from build123d import *

# Parameters (mm, degrees)
SKETCH_1_W          = 45
SKETCH_1_H          = 51
EXTRUDE_1_DEPTH     = 30
SKETCH_2_W          = 27
SKETCH_2_H          = 48
CUT_EXTRUDE_1_DEPTH = 60.793394284
SKETCH_3_R          = 1.5
SKETCH_3_W          = 26
SKETCH_3_H          = 17
CUT_EXTRUDE_2_DEPTH = 61.911821513
FILLET_1_R          = 3
SKETCH_4_R          = 13
SKETCH_4_R_2        = 2
CUT_EXTRUDE_3_DEPTH = 30
FILLET_2_R          = 10
FILLET_3_R          = 5


with BuildPart() as part:
    # 草图1 → 凸台-拉伸1 (new body)
    with BuildSketch(Plane.XY):
        Rectangle(SKETCH_1_W, SKETCH_1_H)
    extrude(amount=EXTRUDE_1_DEPTH)

    # 草图2 → 切除-拉伸1 (cut, through all)
    with BuildSketch(Plane(origin=(22.5, 0, 0), x_dir=(0, 0, -1), z_dir=(1, 0, 0))):
        with Locations((-16.5, 1.5)):
            Rectangle(SKETCH_2_W, SKETCH_2_H)
    extrude(amount=-CUT_EXTRUDE_1_DEPTH, mode=Mode.SUBTRACT)

    # 草图3 → 切除-拉伸2 (cut, through all)
    with BuildSketch(Plane(origin=(0, -22.5, 0), x_dir=(1, 0, 0), z_dir=(0, 1, 0))):
        with Locations(Location((-17.5, -8, 0), (0, 0, 270))):
            Circle(SKETCH_3_R)
        with Locations(Location((-17.5, -25, 0), (0, 0, 270))):
            Circle(SKETCH_3_R)
        with Locations(Location((17.5, -25, 0), (0, 0, 90))):
            Circle(SKETCH_3_R)
        with Locations(Location((17.5, -8, 0), (0, 0, 90))):
            Circle(SKETCH_3_R)
        with Locations((0, -16.5)):
            Rectangle(SKETCH_3_W, SKETCH_3_H)
    extrude(amount=-CUT_EXTRUDE_2_DEPTH, mode=Mode.SUBTRACT)

    # 圆角1
    fillet_1_edges = [part.edges().sort_by_distance(p)[0] for p in [
        (13, -24, 8),
        (13, -24, 25),
        (-13, -24, 25),
        (-13, -24, 8),
    ]]
    fillet(fillet_1_edges, radius=FILLET_1_R)

    # 草图4 → 切除-拉伸3 (cut)
    with BuildSketch(Plane.XY.offset(3)):
        with Locations((0, 3)):
            Circle(SKETCH_4_R)
        with Locations((12.374368671, 15.374368671)):
            Circle(SKETCH_4_R_2)
        with Locations((-12.374368671, 15.374368671)):
            Circle(SKETCH_4_R_2)
        with Locations((-12.374368671, -9.374368671)):
            Circle(SKETCH_4_R_2)
        with Locations((12.374368671, -9.374368671)):
            Circle(SKETCH_4_R_2)
    extrude(amount=-CUT_EXTRUDE_3_DEPTH, mode=Mode.SUBTRACT)

    # 圆角2
    fillet_2_edges = [part.edges().sort_by_distance(p)[0] for p in [
        (-22.5, 25.5, 1.5),
        (22.5, 25.5, 1.5),
    ]]
    fillet(fillet_2_edges, radius=FILLET_2_R)

    # 圆角3
    fillet_3_edges = [part.edges().sort_by_distance(p)[0] for p in [
        (-22.5, -24, 30),
        (22.5, -24, 30),
    ]]
    fillet(fillet_3_edges, radius=FILLET_3_R)


solid = part.part
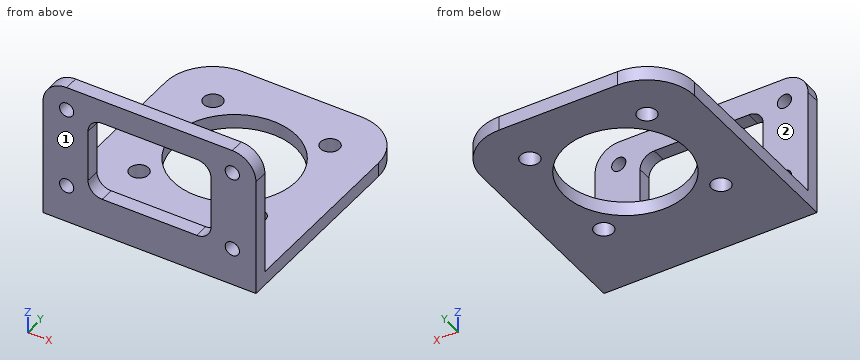
Can you work these out from the model? Positions are in its coordinate system, mm. Face numbers are marked on the shaded views. A direction names the side the tool comes from. Give positions to 0.01 mm unless a question says otherwise; leave off trailing zeros. Order: outer loops, then holes, each group sorted by start corner. A loop starts at its lowest first (then second) coordinate and runs counter-clockwise, first axis right, second up. Notation, with made-up numbers: M 31,16.5 L 83,16.5 A28 ccw 83,37.5 Z; hole C 55.5,24 d2. An arc over 180 degrees is marked long. Use one line per item in the form item = value. Start each with the question number.
Item 1: If we section it at C-C (z = 14.25): Write out the boundary of the cut face in (x, y).
Item 2: If we section it at B-B (y = 8): Write out the boundary of the cut face in (x, z), then the cut area to 3 significant figures.
Item 3: Will these pins go through, and if not, where does the flat tip stop? pin 1 Ø3 at (x, y) = (12.37, 15.37) entering from +Z; pin 2 Ø4 at (x, z) = (17.5, 8) entering from -Y; pin 3 Ø4.5 at (x, y) = (-12.37, 15.37) entering from +Z; pin 4 Ø3.5 at (x, z) = (-17.5, 8) entering from +Y.
Item 4: If I drill on line 1 along Z through (x, y) = (-17, -23); line 2 along Z through (x, y) = (15.5, 4); line 3 along Y through (x, z) = (-15, 14), over which ranges is the centre line in solid material (lowest first)?
Item 5: If we section it at D-D (x = 8.5): Write out the boundary of the cut face in (y, z), then the cut area to 3 significant figures.
Item 6: For the marked faces 1 and 2, which set-ups out of +Z, -Z, +X, -X, +Y, -Y let a thin tool reach every point of the face, with its end or its side?
Item 7: If we section it at A-A (x = 0): Write out the boundary of the cut face in (y, z), then the cut area to 3 significant figures.
Outcome:
q1.outline = M -22.5,-25.5 L -13,-25.5 L -13,-22.5 L -22.5,-22.5 Z; M 13,-25.5 L 22.5,-25.5 L 22.5,-22.5 L 13,-22.5 Z
q2.outline = M -22.5,0 L -12,0 L -12,3 L -22.5,3 Z; M 12,0 L 22.5,0 L 22.5,3 L 12,3 Z
q2.area = 63.0 mm2
q3.pin_1 = through
q3.pin_2 = -25.5
q3.pin_3 = 3
q3.pin_4 = -22.5
q4.line_1 = 0 to 6.59, 9.41 to 23.59, 26.41 to 30
q4.line_2 = 0 to 3
q4.line_3 = -25.5 to -22.5
q5.outline = M -25.5,0 L -6.84,0 L -6.84,3 L -22.5,3 L -22.5,8 L -25.5,8 Z; M -25.5,25 L -22.5,25 L -22.5,30 L -25.5,30 Z; M 12.84,0 L 25.5,0 L 25.5,3 L 12.84,3 Z
q5.area = 124 mm2
q6.face_1 = +Z, -Z, +X, -X, -Y
q6.face_2 = +Z, +X, -X, +Y
q7.outline = M -25.5,0 L -10,0 L -10,3 L -22.5,3 L -22.5,8 L -25.5,8 Z; M -25.5,25 L -22.5,25 L -22.5,30 L -25.5,30 Z; M 16,0 L 25.5,0 L 25.5,3 L 16,3 Z
q7.area = 105 mm2
